The figure shows three views and two pictorial views of one solid part (mm, origin at its lowest corner). Answer the questions. Round coordinates to 2 decimals unless told otherwise and drop trailing zeros. Order: outer loops, then holes, each group sorted by start corner. A loop starts at its lowest first (then second) coordinate and runs counter-clockwise, first axis right, second up.
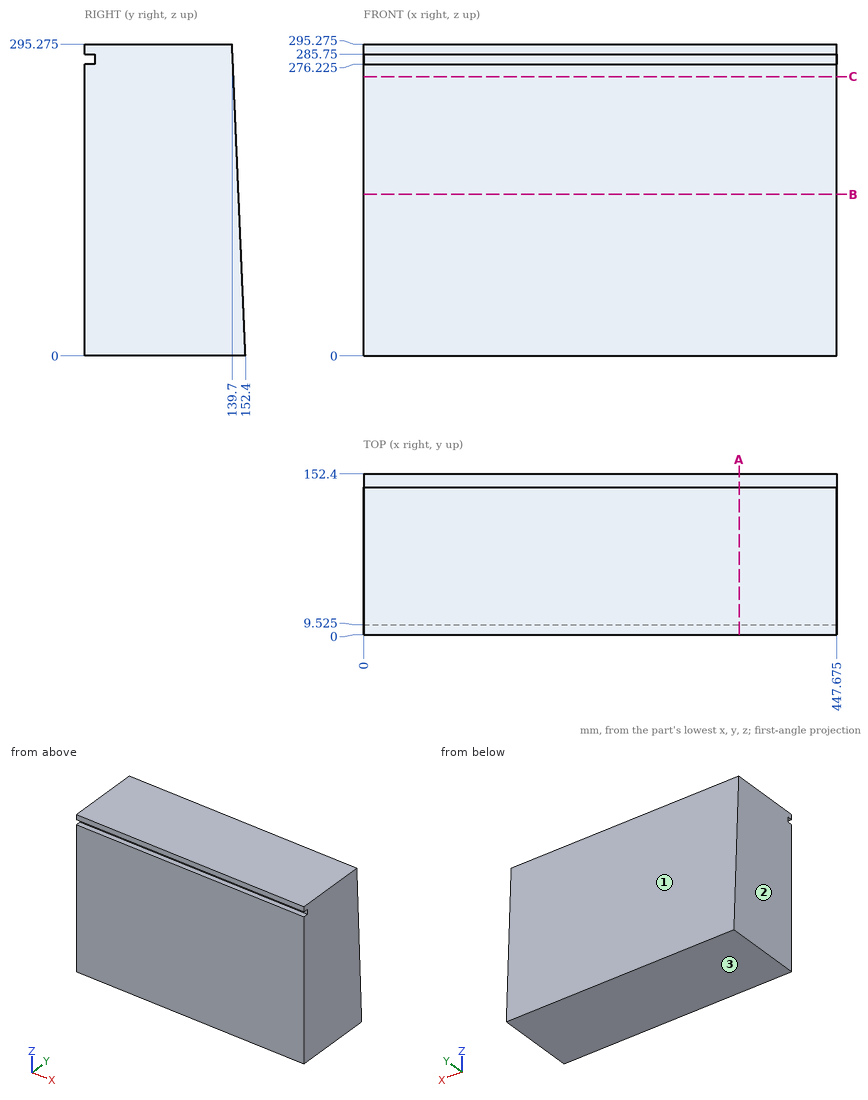
Item 1: Find the intervals of material crossed by line 1 along Y through (x, z) = (375.5, 133); line 2 along Y through (x, z) = (199, 251), in increasing order.
Item 2: For a pull along Z with two mould halves and no side action, classify the marked faces 1, 2 and 3 as released by +Z, released by -Z, zero draft, split by the parting line, or undercut.
Item 3: Find section B-B (z = 153). Write down the section's boundary in (x, y) (3 decimals), plus the area to 3 significant figures.
Item 4: Find section C-C (z = 264.5). Write down the section's boundary in (x, y) (3 decimals).
Item 5: Find section A-A (x = 355.5). Write down the section's boundary in (y, z) (3 decimals), plus the area to 3 significant figures.
Item 6: Given pin 1 (5 mm diameter, centred on x = 245.5, z = 279.5, fed in from -Y) (3 decimals), flat-ended and moving along its own axis, determine where the tip first touches the part or whether it passes through.
Model answer:
1. line 1: y = 0 to 146.68
1. line 2: y = 0 to 141.6
2. face 1: released by +Z
2. face 2: zero draft
2. face 3: released by -Z
3. outline: (0, 0) - (447.675, 0) - (447.675, 145.819) - (0, 145.819) - close
3. area: 65,300 mm2
4. outline: (0, 0) - (447.675, 0) - (447.675, 141.024) - (0, 141.024) - close
5. outline: (0, 0) - (152.4, 0) - (139.7, 295.275) - (0, 295.275) - (0, 285.75) - (9.525, 285.75) - (9.525, 276.225) - (0, 276.225) - close
5. area: 43,000 mm2
6. pin 1: stops at y = 9.525
